Read the model definition and answer for the solid it produces. Units are mm, in the model's axes. A direction names the side the tool comes from. Coordinates: 2 decimals unless noted, no trailing zeros. Order: outer loops, then holes, each group sorted by start corner. A loop starts at its lowest first (then second) coordinate and runs counter-clockwise, first axis right, second up.
Autodesk Fusion 360 part; units mm, degrees
sketch "스케치1" plane through (0, 0, 0) normal (0, 0, 1) x (1, 0, 0)
  line L0 (10, 24) -> (-10, 24)
  line L1 (-10, 24) -> (-10, -24)
  line L2 (-10, -24) -> (10, -24)
  line L3 (10, -24) -> (10, 24)
  line L4 (10, 24) -> (-10, -24) construction
  line L5 (-10, 24) -> (10, -24) construction
  circle A0 centre (0, 0) radius 2.65
  line L6 (0, 0) -> (0, 12)
  circle A1 centre (0, 12) radius 1.6
  line L7 (0, 0) -> (0, -12)
  circle A2 centre (0, -12) radius 1.6
  line L8 (10, 24) -> (11, 24)
  line L9 (11, 24) -> (11, -24)
  line L10 (11, -24) -> (10, -24)
  line L11 (10, -24) -> (10, 24)
  line L12 (11, 24) -> (14, 24)
  line L13 (14, 24) -> (14, -24)
  line L14 (14, -24) -> (11, -24)
  line L15 (11, -24) -> (11, 24)
  line L16 (10, -6) -> (14, -6)
  dimension "d1" = 20
  dimension "d2" = 48
  dimension "d3" = 5.3
  dimension "d4" = 12
  dimension "d5" = 3.2
  dimension "d6" = 12
  dimension "d7" = 3.2
  dimension "d12" = 3
extrude "돌출1" add sketch "스케치1" along normal blind 5 contours L0 L1 L2 L3 L11 | L3 L8 L9 L11 L15 L16
extrude "돌출2" add sketch "스케치1" along normal blind 2.8 contours A2 | A1
extrude "돌출3" add sketch "스케치1" along normal blind 15 contours L9 L12 L13 L15 L16
Q1. The part is cut by section C-C, the plane y = -5. Determine the outline of the cut face in (x, z).
Q2. Each of these flat-tipped pins is pushed along its axis until it touches: P1, Ø8, axis at x = 10, y = -13.5, coming from the +Z side; P2, Ø2, axis at x = 9, y = 4, coming from the -Z side; P3, Ø4.5, axis at x = 12.5, z = 5.5, coming from the -Y side; P4, Ø3, axis at y = 15.5, z = 9.5, coming from the -X side. Where does it stop, or does it pass through?
Q3. The part is cut by section B-B, the plane x = 0. Determine the outline of the cut face in (y, z).
Q4. Straight lines are drawn through the part: L1, parallel to Y at x = 0, z = 3.9; L2, parallel to X at y = -12, z = 3.8; L3, parallel to X at y = 22, z = 13.25. For each, find the intervals that lie inside material, in ascending order.
Q5. The part is cut by section A-A, the plane y = 0. Determine the outline of the cut face in (x, z).
Q6. Determine the mould class of faces 6 (the flat face through (3, 0, 5)), 7 (the cylindrical face through (-0.35, 13.56, 3.88)), 8 (the flat face through (12, -6, 7)), 9 (the flat face through (0, -12, 2.8)) for opening direction Y: +Y half, -Y half, draft (parallel to the pull), parting line (faces both ways), or undercut.
Q7. The part is cut by section D-D, the plane z = 7.25. Determine the outline of the cut face in (x, y), then the cut area to 3 significant figures.
Q8. Which of the six approach directions +Z, -Z, +X, -X, +Y, -Y give full straight-line access (tool end or side, diameter ignored) to faces 1 (the flat face through (4, 24, 4)), 2 (the flat face through (11, 9, 10)), 3 (the flat face through (10, -15, 2)), 4 (the flat face through (0, 12, 2.8)), 5 (the flat face through (14, 9, 7))?
Computed values:
1. outline: (-10, 0) - (14, 0) - (14, 15) - (11, 15) - (11, 5) - (-10, 5) - close
2. P1: stops at z = 5
2. P2: stops at z = 0
2. P3: stops at y = -6
2. P4: stops at x = 11
3. outline: (-24, 0) - (-2.65, 0) - (-2.65, 5) - (-10.4, 5) - (-10.4, 2.8) - (-13.6, 2.8) - (-13.6, 5) - (-24, 5) - close; (2.65, 0) - (24, 0) - (24, 5) - (13.6, 5) - (13.6, 2.8) - (10.4, 2.8) - (10.4, 5) - (2.65, 5) - close
4. L1: y = -24 to -13.6, -10.4 to -2.65, 2.65 to 10.4, 13.6 to 24
4. L2: x = -10 to -1.6, 1.6 to 10
4. L3: x = 11 to 14
5. outline: (-10, 0) - (-2.65, 0) - (-2.65, 5) - (-10, 5) - close; (2.65, 0) - (14, 0) - (14, 15) - (11, 15) - (11, 5) - (2.65, 5) - close
6. face 6: draft
6. face 7: undercut
6. face 8: -Y half
6. face 9: undercut
7. outline: (11, -6) - (14, -6) - (14, 24) - (11, 24) - close
7. area: 90.0 mm2
8. face 1: +Z, -Z, +X, -X, +Y
8. face 2: +Z, -X, +Y, -Y
8. face 3: +Z, -Z, +X, -Y
8. face 4: +Z
8. face 5: +Z, -Z, +X, +Y, -Y
